```python
from build123d import *

# Parameters (mm, degrees)
SKETCH1_W               = 25
SKETCH1_H               = 20
SKETCH1_R               = 2
BASE_FLANGE1_DEPTH      = 3
EDGE_FLANGE1_DEPTH      = 25
EDGE_FLANGE1_START      = 3
EDGE_FLANGE1_PROFILE_W  = 25
EDGE_FLANGE1_PROFILE_H  = 22.976474449
EDGE_FLANGE1_PROFILE_R  = 2
EDGE_FLANGE1_FLAT_DEPTH = 3


# Sheet-metal steps are written as plain solids
with BuildPart() as part:
    # Sketch1 → Base-Flange1 (new body)
    with BuildSketch(Plane.XY):
        with Locations((7.971698113, 5.754716981)):
            Rectangle(SKETCH1_W, SKETCH1_H)
        with Locations((7.971698113, 4.754716981)):
            Circle(SKETCH1_R, mode=Mode.SUBTRACT)
    extrude(amount=-BASE_FLANGE1_DEPTH)

    # Edge-Flange1 bend section (across the edge) → Edge-Flange1 (add)
    with BuildSketch(Plane(origin=(20.471698113, 17.778242532, 0), x_dir=(0, -0.9271838545667858, 0.3746065934159162), z_dir=(-1, 0, 0))):
        with BuildLine():
            Line((-3, 2.023525551), (0, 2.023525551))
            ThreePointArc((0, 2.023525551), (0.512887282, 0.34594684), (1.87618022, -0.758026013))
            Line((1.87618022, -0.758026013), (0.75236044, -3.539577577))
            ThreePointArc((0.75236044, -3.539577577), (-1.974225435, -1.33163187), (-3, 2.023525551))
        make_face()
    extrude(amount=EDGE_FLANGE1_DEPTH)

    # Edge-Flange1 profile (on flange) → Edge-Flange1 flat (add)
    with BuildSketch(Plane(origin=(0, 17.778242532, 0), x_dir=(-1, 0, 0), z_dir=(0, 0.9271838545667858, -0.3746065934159162)).offset(EDGE_FLANGE1_START)):
        with Locations((-7.971698113, 13.511762775)):
            Rectangle(EDGE_FLANGE1_PROFILE_W, EDGE_FLANGE1_PROFILE_H)
        with Locations((-7.971698113, 18)):
            Circle(EDGE_FLANGE1_PROFILE_R, mode=Mode.SUBTRACT)
    extrude(amount=-EDGE_FLANGE1_FLAT_DEPTH)


solid = part.part
```
Geometry check sheet. Reference: the model listing, model coordinates, mm. A direction names the side the tool comes from. Round coordinates to 2 decimals unless told otherwise and drop trailing zeros. Loops run counter-clockwise (first coordinate to the right, second up) from the corner with the lowest first, then second, coordinate; pieces in that order, holes last. Notation, with made-up numbers: (-5.5, -11.5) - (52.5, -11.5) arc R14 ccw to (52.5, 4.5) - close; hole circle Ø1 at (9.25, 53). An arc over 180 degrees is marked (long way). Use a Markdown table: item, result.
Q1. Go/stop test with flat-tipped pins: P1, Ø6.5, axis at x = 7.97, y = 4.75, coming from the +Z side; P2, Ø1.5, axis at x = 10.5, y = 17.5, coming from the +Z side; P3, Ø5, axis at x = 12, z = 15, coming from the +Y side. Record where each tip stops, or that it passes through.
Solutions:
| item | result |
|---|---|
| P1 | stops at z = 0 |
| P2 | stops at z = 1.33 |
| P3 | stops at y = 28.08 |
Q2. Cross-section at C-C on y = 0. Record the cut outline in (x, z).
Solutions:
| item | result |
|---|---|
| outline | (-4.53, -3) - (20.47, -3) - (20.47, 0) - (-4.53, 0) - close |
Q3. Access from +Z, -Z, +X, -X, +Y, -Y to the whole of each face (thin tool, end or side, straight path). Record for faces 1 (the flat face through (8.15, 28.55, 22.61)), 2 (the flat face through (8, 8, 0)).
Solutions:
| item | result |
|---|---|
| face 1 | +Z, +X, -X, +Y |
| face 2 | +Z, +X, -X, -Y |
Q4. Cross-section at D-D on z = -0.75. Record the cut outline in (x, y).
Solutions:
| item | result |
|---|---|
| outline | (-4.53, -4.25) - (20.47, -4.25) - (20.47, 20.44) - (-4.53, 20.44) - close; hole circle Ø4 at (7.97, 4.75) |
Q5. Cross-section at A-A on x = 16.25. Record the cut outline in (y, z), plus the area to 3 significant figures.
Solutions:
| item | result |
|---|---|
| outline | (-4.25, -3) - (15.75, -3) arc R6 ccw to (21.32, 0.75) - (29.92, 22.06) - (27.14, 23.18) - (18.54, 1.88) arc R3 cw to (15.75, 0) - (-4.25, 0) - close |
| area | 145 mm2 |
Q6. Material ranges on line 1 (Z direction, x = -2.75, y = 1.5); line 2 (Y direction, x = 12.25, z = 18.5); line 3 (Y direction, x = 0, z = 15.5), recorded low to high.
Solutions:
| item | result |
|---|---|
| line 1 | z = -3 to 0 |
| line 2 | y = 25.25 to 28.49 |
| line 3 | y = 24.04 to 27.28 |
Q7. Draft check along Y on faces 3 (the cylindrical face through (5.974, 4.843, -1.479)), 4 (the cylindrical face through (8.147, 17.453, 0.527)), 5 (the flat face through (-4.528, 21, 5)), 6 (the cylindrical face through (8.15, 19.07, -2)). Enter one of: released by +Y, released by -Y, zero draft, split by the parting line, or undercut.
Solutions:
| item | result |
|---|---|
| face 3 | undercut |
| face 4 | released by -Y |
| face 5 | zero draft |
| face 6 | released by +Y |
Q8. Cross-section at B-B on x = 7. Record the cut outline in (y, z).
Solutions:
| item | result |
|---|---|
| outline | (-4.25, -3) - (3.01, -3) - (3.01, 0) - (-4.25, 0) - close; (6.5, -3) - (15.75, -3) arc R6 ccw to (21.32, 0.75) - (26.65, 13.94) - (23.87, 15.07) - (18.54, 1.88) arc R3 cw to (15.75, 0) - (6.5, 0) - close; (25.18, 18.31) - (27.96, 17.19) - (29.92, 22.06) - (27.14, 23.18) - close |
